```python
from build123d import *

# Parameters (mm, degrees)
F1_DEPTH = 3.175
F2_R     = 5.08
F3_R     = 5.08


# Not quite as in the source:
# - a feature names something its author has since deleted; it is built from what else it names


with BuildPart() as f1:
    # F0 (on Front) → F1 (new body)
    with BuildSketch(Plane.XZ):
        Polygon((45.1797973156, 19.05), (-107.2202026844, 19.05), (-107.2202026844, -31.75), (-81.8202026844, -31.75), (-81.8202026844, -19.05), (-31.0202026844, 6.35), (19.7797973156, -19.05), (19.7797973156, -31.75), (45.1797973156, -31.75), (45.1797973156, -6.35), align=None)
    extrude(amount=F1_DEPTH)

    # F2
    f2_edges = [f1.edges().sort_by_distance(p)[0] for p in [
        (-81.820203, -1.5875, -19.05),
    ]]
    fillet(f2_edges, radius=F2_R)

    # F3
    f3_edges = [f1.edges().sort_by_distance(p)[0] for p in [
        (-81.820203, -1.5875, -31.75),
        (19.779797, -1.5875, -31.75),
    ]]
    fillet(f3_edges, radius=F3_R)


solid = f1.part
```
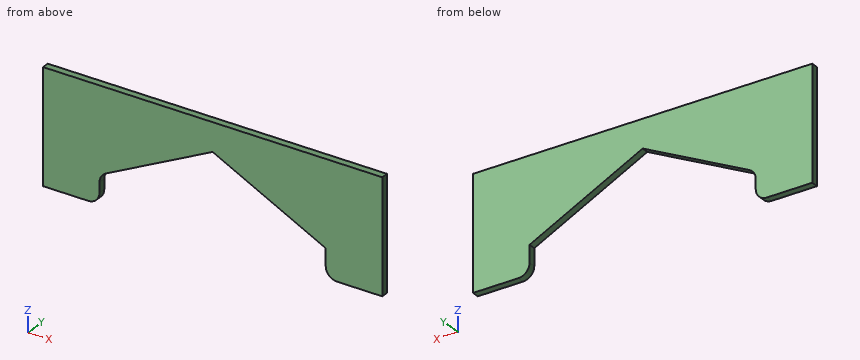
For this review, take the finished solid that the model builds, in its own axes (mm). Give positions to 0.01 mm unless a question says otherwise; leave off trailing zeros. Loops run counter-clockwise (first coordinate to the right, second up) from the corner with the lowest first, then second, coordinate; pieces in that order, holes last. Notation, with made-up numbers: M 88,56 L 95,56 A21 ccw 95,94 Z; hole C -5.5,22 d8. An arc over 180 degrees is marked long. One line per item, written item: value. Start each with the question number.
Q1. Add section C-C (x = -40). Give the boundary of the cut face in (y, z) (3 decimals).
Q2. Add section B-B (y = -0.95). Give the boundary of the cut face in (x, z).
Q3. Clearance check with a flat-ended pin moving along its axis: pin 1 Ø1 at (x, y) = (-79, -2) entering from -Z. State where the tip first meets the part, or that it passes through.
Q4. Add section A-A (z = -3.5). Give the boundary of the cut face in (x, y) (3 decimals).
Q5. For L1, parallel to X at y = -0.55, z = -24.5; L2, parallel to X at y = -1.85, z = -20.5; L3, parallel to Z at x = -4.5, y = -1.95, list the stretches that pass through material, from the lowest coordinate up.
Q6. Add section D-D (x = -60). Give the boundary of the cut face in (y, z) (3 decimals), and give its area (3 significant figures).
Reply:
1. outline: M -3.175,1.86 L 0,1.86 L 0,19.05 L -3.175,19.05 Z
2. outline: M -107.22,-31.75 L -86.9,-31.75 A5.08 ccw -81.82,-26.67 L -81.82,-22.19 A5.08 cw -79.01,-17.65 L -31.02,6.35 L 19.78,-19.05 L 19.78,-26.67 A5.08 ccw 24.86,-31.75 L 45.18,-31.75 L 45.18,19.05 L -107.22,19.05 Z
3. pin 1: z = -17.92
4. outline: M -107.22,-3.175 L -50.72,-3.175 L -50.72,0 L -107.22,0 Z; M -11.32,-3.175 L 45.18,-3.175 L 45.18,0 L -11.32,0 Z
5. L1: -107.22 to -81.82, 19.78 to 45.18
5. L2: -107.22 to -81.53, 19.78 to 45.18
5. L3: -6.91 to 19.05
6. outline: M -3.175,-8.14 L 0,-8.14 L 0,19.05 L -3.175,19.05 Z
6. area: 86.3 mm²
